```python
from build123d import *

# Parameters (mm, degrees)
F3_W      = 50.8
F3_H      = 50.8
F4_DEPTH  = 25.4
F4_FACE_W = 50.8
F4_FACE_H = 50.8
F5_DEPTH  = 25.4
F6_W      = 38.1
F6_H      = 12.7
F7_DEPTH  = 76.2
F8_W      = 12.7
F8_H      = 19.05
F9_DEPTH  = 76.2
F11_DEPTH = 76.2


with BuildPart() as f4:
    # F3 (on Front) → F4 (new body)
    with BuildSketch(Plane.XZ):
        Rectangle(F3_W, F3_H)
    extrude(amount=F4_DEPTH)

    # F4_face (on face) → F5 (join)
    with BuildSketch(Plane(origin=(0, 0, 0), x_dir=(1, 0, 0), z_dir=(0, 1, 0))):
        Rectangle(F4_FACE_W, F4_FACE_H)
    extrude(amount=F5_DEPTH)

    # F6 (on offset) → F7 (cut)
    with BuildSketch(Plane.XZ.offset(50.8)):
        with Locations((6.35, 12.7)):
            Rectangle(F6_W, F6_H)
        with Locations((-6.35, -12.7)):
            Rectangle(F6_W, F6_H)
    extrude(amount=-F7_DEPTH, mode=Mode.SUBTRACT)

    # F8 (on offset) → F9 (cut)
    with BuildSketch(Plane.YZ.offset(50.8)):
        with Locations((0, 15.875)):
            Rectangle(F8_W, F8_H)
        with Locations((0, -15.875)):
            Rectangle(F8_W, F8_H)
    extrude(amount=-F9_DEPTH, mode=Mode.SUBTRACT)

    # F10 (on offset) → F11 (cut)
    with BuildSketch(Plane.XY.offset(50.8)):
        Polygon((25.4, -6.35), (25.4, 6.35), (12.7, 0), align=None)
        Polygon((0, 9.817213), (-25.4, 12.992213), (-25.4, -12.633159), (0, -9.232787), (-12.7, -2.882787), (-12.7, 3.467213), align=None)
    extrude(amount=-F11_DEPTH, mode=Mode.SUBTRACT)


solid = f4.part
```
Input: part model. Units: mm. Frame: model coordinates. A direction names the side the tool comes from. Round coordinates to 2 decimals unless told otherwise and drop trailing zeros. Loops run counter-clockwise (first coordinate to the right, second up) from the corner with the lowest first, then second, coordinate; pieces in that order, holes last. Notation, with made-up numbers: (83.5, 57.5) -> (107.5, 57.5) arc R20 cw to (107.5, 64.5) -> close; hole circle Ø9 at (15, 34). An arc over 180 degrees is marked (long way). Write each question's results on one line, items separated by ' | '.
1. Ray query, line 1 (Z direction, x = 1, y = 15.5); line 2 (Z direction, x = -15.5, y = 14); line 3 (Y direction, x = 12.5, z = -20.5). Return the intervals inside material, ascending. Write a range as from..to.
Geometry results:
line 1: -25.4..-19.05, -6.35..6.35, 19.05..25.4 | line 2: -25.4..-19.05, -6.35..25.4 | line 3: -25.4..-6.35, 6.35..25.4
2. Section D-D (x = -8). Return loops of the section in (y, z).
Geometry results:
outline: (-25.4, -25.4) -> (-10.3, -25.4) -> (-10.3, -19.05) -> (-25.4, -19.05) -> close; (-25.4, -6.35) -> (-10.3, -6.35) -> (-10.3, 6.35) -> (-25.4, 6.35) -> close; (-25.4, 19.05) -> (-10.3, 19.05) -> (-10.3, 25.4) -> (-25.4, 25.4) -> close; (-5.23, -6.35) -> (5.82, -6.35) -> (5.82, 6.35) -> (-5.23, 6.35) -> close; (10.82, -25.4) -> (25.4, -25.4) -> (25.4, -19.05) -> (10.82, -19.05) -> close; (10.82, -6.35) -> (25.4, -6.35) -> (25.4, 6.35) -> (10.82, 6.35) -> close; (10.82, 19.05) -> (25.4, 19.05) -> (25.4, 25.4) -> (10.82, 25.4) -> close
3. Section C-C (y = 18). Return loops of the section in (x, z), and give its area (3 significant figures).
Geometry results:
outline: (-25.4, -25.4) -> (25.4, -25.4) -> (25.4, 6.35) -> (-12.7, 6.35) -> (-12.7, 19.05) -> (25.4, 19.05) -> (25.4, 25.4) -> (-25.4, 25.4) -> (-25.4, -6.35) -> (12.7, -6.35) -> (12.7, -19.05) -> (-25.4, -19.05) -> close | area: 1,610 mm2
4. First-contact query: P1, Ø10, axis at y = 13.5, z = -14.5, coming from the -X side; P2, Ø6.5, axis at y = -15, z = 12.5, coming from the +X side; P3, Ø6.5, axis at y = -18.5, z = -12, coming from the -X side; P4, Ø5, axis at y = -1.5, z = 3, coming from the -X side. Flat tips, straight axial feed; report the tip coordinate or a pass-through.
Geometry results:
P1: x = -25.4 | P2: x = -12.7 | P3: x = 12.7 | P4: x = -12.7
5. Set-up query: faces 1 (the face through (10, -6.35, 22)), 2 (the face through (-15.344, 11.735, 9.747)), 3 (the face through (6, 16, 19.05)), 4 (the face through (12.7, 16, -13)). Return all of +Z, -Z, +X, -X, +Y, -Y with unobstructed straight access to the full face (end or side cutting, diameter ignored); none if empty.
Geometry results:
face 1: +Z, +X, -X | face 2: +Z, -Z, -X | face 3: +X, +Y, -Y | face 4: -X, +Y, -Y
6. Mould query, pull axis Y, two halves, no side actions, for faces 5 (the face through (0, -25.4, 0)), 6 (the face through (-25.4, 19, -22)), 7 (the face through (-3.516, 8.059, 22.269)), 8 (the face through (18.96, -3.13, 0.09)). Classes: +Y half, -Y half, draft (parallel to the pull), parting line (faces both ways), or undercut.
Geometry results:
face 5: -Y half | face 6: draft | face 7: undercut | face 8: undercut
7. Section B-B (x = 6). Return loops of the section in (y, z), and give its area (3 significant figures).
Geometry results:
outline: (-25.4, -25.4) -> (-6.35, -25.4) -> (-6.35, -19.05) -> (-25.4, -19.05) -> close; (-25.4, -6.35) -> (25.4, -6.35) -> (25.4, 6.35) -> (-25.4, 6.35) -> close; (-25.4, 19.05) -> (-6.35, 19.05) -> (-6.35, 25.4) -> (-25.4, 25.4) -> close; (6.35, -25.4) -> (25.4, -25.4) -> (25.4, -19.05) -> (6.35, -19.05) -> close; (6.35, 19.05) -> (25.4, 19.05) -> (25.4, 25.4) -> (6.35, 25.4) -> close | area: 1,130 mm2
8. Section A-A (z = 13). Return loops of the section in (x, y).
Geometry results:
outline: (-25.4, -25.4) -> (-12.7, -25.4) -> (-12.7, -10.93) -> (-25.4, -12.63) -> close; (-25.4, 12.99) -> (-12.7, 11.4) -> (-12.7, 25.4) -> (-25.4, 25.4) -> close
